Work out the finished part from the listing and answer in its coordinate system (mm). Round coordinates to 2 decimals unless told otherwise and drop trailing zeros. Loops run counter-clockwise (first coordinate to the right, second up) from the corner with the lowest first, then second, coordinate; pieces in that order, holes last. Notation, with made-up numbers: (64.25, 12) - (79.25, 12) arc R24 ccw to (79.25, 37) - close; hole circle Ø6 at (13, 57). An arc over 180 degrees is marked (long way). Return JSON: item names as keys, results as strings.
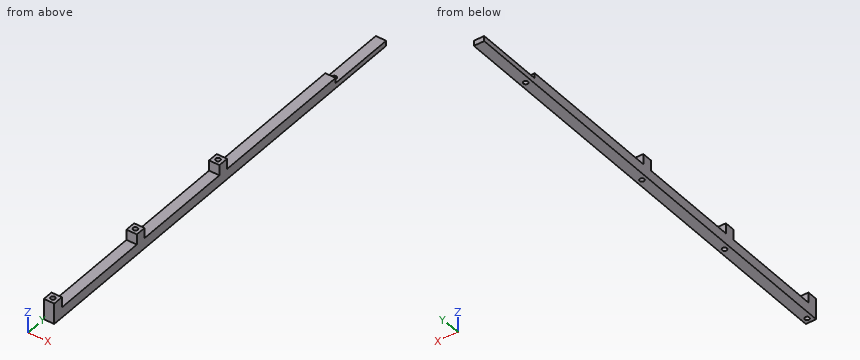
from build123d import *

# Parameters (mm, degrees)
SKETCH1_W                  = 6.35
SKETCH1_H                  = 12.7
BOSS_EXTRUDE1_DEPTH        = 275.59
CUT_EXTRUDE_THIN1_DEPTH    = 276.955540984
F_35_0_11_DIAMETER_HOLE1_D = 2.794


with BuildPart() as part:
    # Sketch1 → Boss-Extrude1 (new body)
    with BuildSketch(Plane(origin=(0, 0, 0), x_dir=(1, 0, 0), z_dir=(0, 1, 0))):
        with Locations((3.175, 6.35)):
            Rectangle(SKETCH1_W, SKETCH1_H)
    extrude(amount=BOSS_EXTRUDE1_DEPTH)

    # Sketch2 → Cut-Extrude-Thin1 (cut, through all)
    with BuildSketch(Plane.ZY):
        Polygon((0, 233.68), (-9.525, 233.68), (-9.525, 275.59), (-9.52510033, 275.59), (-9.52510033, 233.67989967), (0, 233.67989967), align=None)
        Polygon((0, 143.51), (-6.35, 143.51), (-6.35, 233.68), (-6.35010033, 233.68), (-6.35010033, 143.50989967), (0, 143.50989967), align=None)
        Polygon((0, 137.16), (-6.35, 137.16), (-6.35, 74.93), (0, 74.93), (0, 74.93010033), (-6.34989967, 74.93010033), (-6.34989967, 137.15989967), (0, 137.15989967), align=None)
        Polygon((0, 68.58), (-6.35, 68.58), (-6.35, 6.35), (0, 6.35), (0, 6.35010033), (-6.34989967, 6.35010033), (-6.34989967, 68.57989967), (0, 68.57989967), align=None)
    extrude(amount=-CUT_EXTRUDE_THIN1_DEPTH, mode=Mode.SUBTRACT)


with BuildPart() as cut_extrude_thin1_kept_piece:
    # of the separate pieces the step leaves, the one the design keeps (cut_extrude_thin1_pieces_kept)
    add(part.part.solids().sort_by_distance((0, 0, 0))[0])

    # #35 (0.11) Diameter Hole1 (through all)
    with Locations(Plane.XY):
        with Locations((3.175, 236.855), (3.175, 140.335), (3.175, 71.755), (3.175, 3.175)):
            Hole(F_35_0_11_DIAMETER_HOLE1_D / 2)


solid = cut_extrude_thin1_kept_piece.part
1) Section C-C (y = 201.5) is taken. Give the vertices of the cut face in (x, z).
Verdict:
{"outline": "(0, -12.7) - (6.35, -12.7) - (6.35, -6.35) - (0, -6.35) - close"}
2) Section A-A (z = -3) is taken. Give the vertices of the cut face in (x, y) (3 decimals), and give its area (3 significant figures).
Verdict:
{"outline": "(0, 0) - (6.35, 0) - (6.35, 6.35) - (0, 6.35) - close; (0, 68.58) - (6.35, 68.58) - (6.35, 74.93) - (0, 74.93) - close; (0, 137.16) - (6.35, 137.16) - (6.35, 143.51) - (0, 143.51) - close; hole circle Ø2.794 at (3.175, 3.175); hole circle Ø2.794 at (3.175, 71.755); hole circle Ø2.794 at (3.175, 140.335)", "area": "103 mm2"}
3) Section B-B (x = 3.5) is taken. Count the separate pieces of the cut face and the enclosed holes in it, and give its area (3 significant figures).
Verdict:
{"separate pieces": "5", "enclosed holes": "0", "area": "1,630 mm2"}
4) Section D-D (y = 259.5) is taken. Give the vertices of the cut face in (x, z).
Verdict:
{"outline": "(0, -12.7) - (6.35, -12.7) - (6.35, -9.53) - (0, -9.53) - close"}
5) Flat-ended cylindrical pins translate along their axes: pin 1 (3 mm diameter, centred on x = 3.5, y = 46.5, fed in from +Z); pin 2 (1.9 mm diameter, centred on x = 3, z = -4.5, fed in from +Y); pin 3 (2.5 mm diameter, centred on x = 4, z = -8, fed in from +Y). Find the tip coordinate at first contact, or state that the pin passes through.
Verdict:
{"pin 1": "stops at z = -6.35", "pin 2": "stops at y = 143.51", "pin 3": "stops at y = 233.68"}
6) Find the intervals of material crossed by L1, parallel to Y at x = 4.75, z = -2.5; L2, parallel to Y at x = 3, z = -8.25; L3, parallel to Y at x = 3.25, z = -2.25, in increasing order.
Verdict:
{"L1": "y = 0 to 6.35, 68.58 to 74.93, 137.16 to 143.51", "L2": "y = 0 to 1.79, 4.56 to 70.37, 73.14 to 138.95, 141.72 to 233.68", "L3": "y = 0 to 1.78, 4.57 to 6.35, 68.58 to 70.36, 73.15 to 74.93, 137.16 to 138.94, 141.73 to 143.51"}
